from build123d import *

# Parameters (mm, degrees)
SKETCH_1_W          = 14
SKETCH_1_H          = 12
EXTRUDE_1_DEPTH     = 9
FILLET_2_R          = 1
FILLET_3_R          = 1
SKETCH_8_W          = 10
SKETCH_8_H          = 5.607572988
CUT_EXTRUDE_2_DEPTH = 10
SKETCH_9_W          = 10
SKETCH_9_H          = 6
EXTRUDE_3_DEPTH     = 10.1
SKETCH_10_R         = 1.75
CUT_EXTRUDE_3_DEPTH = 0.5
CUT_EXTRUDE_4_DEPTH = 22.740745157
SKETCH_12_W         = 4
SKETCH_12_H         = 5
CUT_EXTRUDE_5_DEPTH = 5
EXTRUDE_5_DEPTH     = 3
SKETCH_17_R         = 5
EXTRUDE_6_DEPTH     = 7
SKETCH_14_R         = 3.5
SKETCH_14_R_2       = 3
EXTRUDE_7_DEPTH     = 10
FILLET_5_R          = 0.5
CUT_EXTRUDE_START   = -5
SKETCH_18_R         = 3
CUT_EXTRUDE_7_DEPTH = 5
FILLET_6_R          = 0.5


# Some blends are built 0.0001 mm under size
with BuildPart() as part:
    # 草图1 → 凸台-拉伸1 (new body)
    with BuildSketch(Plane(origin=(0, 0, 0), x_dir=(1, 0, 0), z_dir=(0, 1, 0))):
        with Locations((7, 6)):
            Rectangle(SKETCH_1_W, SKETCH_1_H)
    extrude(amount=EXTRUDE_1_DEPTH)

    # 圆角2
    fillet_2_edges = [part.edges().sort_by_distance(p)[0] for p in [
        (14, 9, -6),
        (7, 9, -12),
        (0, 9, -6),
        (7, 9, 0),
    ]]
    fillet(fillet_2_edges, radius=FILLET_2_R)

    # 草图4 → 放样1 section 0
    with BuildSketch(Plane.XZ):
        with BuildLine():
            Line((0, 0), (14, 0))
            Line((14, 0), (14, -12))
            Line((14, -12), (0, -12))
            Line((0, -12), (0, 0))
        make_face()
    # 草图5 → 放样1 section 1
    with BuildSketch(Plane(origin=(0, -11, 0), x_dir=(-1, 0, 0), z_dir=(0, -1, 0))):
        with BuildLine():
            Line((-2, 1), (-12, 1))
            Line((-12, 1), (-12, 11))
            Line((-12, 11), (-2, 11))
            Line((-2, 11), (-2, 1))
        make_face()
    loft()

    # 圆角3
    # the kernel refuses this fillet: 1 mm, written as the material it takes off along each edge
    with BuildSketch(Plane(origin=(14.438278825, 2.410533539, -12.219139413), x_dir=(0.015936381457793344, 0.08765009801785527, 0.9960238411119947), z_dir=(-0.1781741612749496, -0.9799578870122228, 0.0890870806374748)), Plane(origin=(14.438278825, 2.410533539, 0.219139413), x_dir=(-0.9839989676081822, 0.17744243678180333, 0.016131130616527562), z_dir=(-0.1781741612749496, -0.9799578870122228, -0.08908708063747467))) as fillet_3_piece_1:
        with BuildLine():
            CenterArc((FILLET_3_R * 0.983933522321, FILLET_3_R), FILLET_3_R, 180.927975892, 89.072024108)
            Line((-FILLET_3_R * 0.0159353215369, FILLET_3_R * 0.983804473396), (0, 0))
            Line((0, 0), (FILLET_3_R * 0.983933522321, 0))
        make_face()
    extrude(amount=16.144639772, mode=Mode.SUBTRACT)
    with BuildSketch(Plane(origin=(-0.438278825, 2.410533539, -12.219139413), x_dir=(-0.015936381457791863, 0.08765009801785537, 0.9960238411119947), z_dir=(0.1781741612749496, -0.9799578870122228, 0.08908708063747463)), Plane(origin=(-0.438278825, 2.410533539, 0.219139413), x_dir=(0.9839989676081822, 0.17744243678180333, 0.016131130616527607), z_dir=(0.1781741612749496, -0.9799578870122228, -0.0890870806374748))) as fillet_3_piece_2:
        with BuildLine():
            CenterArc((FILLET_3_R * 0.983933522321, -FILLET_3_R), FILLET_3_R, 90, 89.072024108)
            Line((-FILLET_3_R * 0.0159353215369, -FILLET_3_R * 0.983804473396), (0, 0))
            Line((0, 0), (FILLET_3_R * 0.983933522321, 0))
        make_face()
    extrude(amount=16.144639772, mode=Mode.SUBTRACT)

    # 草图8 → 切除-拉伸2 (cut)
    with BuildSketch(Plane(origin=(0, 0, -12), x_dir=(-1, 0, 0), z_dir=(0, 0, -1))):
        with Locations((-7, 10.303786494)):
            Rectangle(SKETCH_8_W, SKETCH_8_H)
    extrude(amount=-CUT_EXTRUDE_2_DEPTH, mode=Mode.SUBTRACT)

    # 草图9 → 凸台-拉伸3 (add)
    with BuildSketch(Plane(origin=(0, 0, -2), x_dir=(-1, 0, 0), z_dir=(0, 0, -1))):
        with Locations((-7, 10.5)):
            Rectangle(SKETCH_9_W, SKETCH_9_H)
    extrude(amount=EXTRUDE_3_DEPTH)

    # 草图10 → 切除-拉伸3 (cut)
    with BuildSketch(Plane(origin=(0, 0, -12.1), x_dir=(-1, 0, 0), z_dir=(0, 0, -1))):
        with Locations((-4.5, 10)):
            Circle(SKETCH_10_R)
        with Locations((-9.5, 10)):
            Circle(SKETCH_10_R)
    extrude(amount=-CUT_EXTRUDE_3_DEPTH, mode=Mode.SUBTRACT)

    # 草图11 → 切除-拉伸4 (cut, through all)
    with BuildSketch(Plane.ZY.offset(-2)):
        Polygon((-12.1, 12.5), (-12.1, 13.5), (-9.1, 13.5), align=None)
    extrude(amount=-CUT_EXTRUDE_4_DEPTH, mode=Mode.SUBTRACT)

    # 草图12 → 切除-拉伸5 (cut)
    with BuildSketch(Plane(origin=(0, 13.5, 0), x_dir=(1, 0, 0), z_dir=(0, 1, 0))):
        with Locations((4.5, 5.1)):
            Rectangle(SKETCH_12_W, SKETCH_12_H)
        with Locations((9.5, 5.1)):
            Rectangle(SKETCH_12_W, SKETCH_12_H)
    extrude(amount=-CUT_EXTRUDE_5_DEPTH, mode=Mode.SUBTRACT)

    # 草图15 → 凸台-拉伸5 (add)
    with BuildSketch(Plane.XZ.offset(11)):
        with BuildLine():
            Line((6.95, -5.251668523), (6.95, -6.748331477))
            ThreePointArc((6.95, -6.748331477), (6.25, -6), (6.95, -5.251668523))
        make_face()
        with BuildLine():
            Line((7.05, -5.251668523), (7.05, -6.748331477))
            ThreePointArc((7.05, -6.748331477), (7.75, -6), (7.05, -5.251668523))
        make_face()
    extrude(amount=EXTRUDE_5_DEPTH)

    # 草图17 → 凸台-拉伸6 (add)
    with BuildSketch(Plane.XZ.offset(11)):
        with Locations(Location((7, -6, 0), (0, 0, 270))):
            Circle(SKETCH_17_R)
    extrude(amount=EXTRUDE_6_DEPTH)

    # 草图14 → 凸台-拉伸7 (add)
    with BuildSketch(Plane.XZ.offset(11)):
        with Locations(Location((7, -6, 0), (0, 0, 270))):
            Circle(SKETCH_14_R)
        with Locations(Location((7, -6, 0), (0, 0, 270))):
            Circle(SKETCH_14_R_2, mode=Mode.SUBTRACT)
    extrude(amount=EXTRUDE_7_DEPTH)

    # 圆角5
    fillet_5_edges = [part.edges().sort_by_distance(p)[0] for p in [
        (7, -21, -2.5),
    ]]
    fillet(fillet_5_edges, radius=FILLET_5_R - 0.0001)  # a hair under: the kernel refuses the full size

    # 草图18 → 切除-拉伸7 (cut)
    with BuildSketch(Plane.XZ.offset(18).offset(CUT_EXTRUDE_START)):
        with Locations(Location((7, -6, 0), (0, 0, 270))):
            Circle(SKETCH_18_R)
        with BuildLine():
            Line((6.357738371, -5.9), (7.642261629, -5.9))
            ThreePointArc((7.642261629, -5.9), (7, -5.35), (6.357738371, -5.9))
        make_face(mode=Mode.SUBTRACT)
        with BuildLine():
            Line((6.357738371, -6.1), (7.642261629, -6.1))
            ThreePointArc((7.642261629, -6.1), (7, -6.65), (6.357738371, -6.1))
        make_face(mode=Mode.SUBTRACT)
    extrude(amount=CUT_EXTRUDE_7_DEPTH, mode=Mode.SUBTRACT)

    # 圆角6
    fillet_6_edges = [part.edges().sort_by_distance(p)[0] for p in [
        (7, -18, -5.35),
        (7, -18, -6.65),
    ]]
    fillet(fillet_6_edges, radius=FILLET_6_R)


solid = part.part
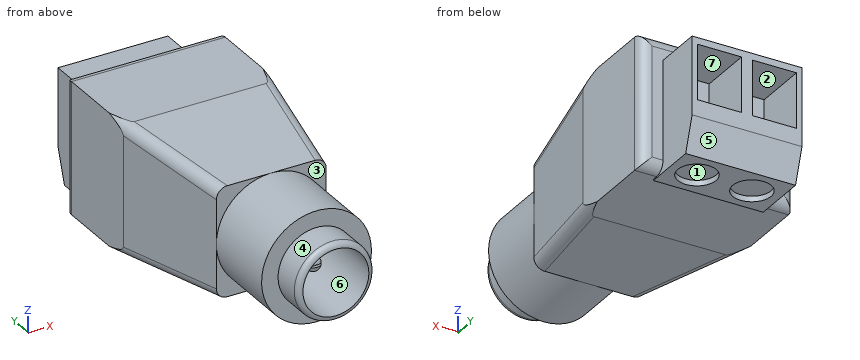
CAD build for the part. Positions are in the model's coordinates, mm. Face numbers are marked on the shaded views. A direction names the side the tool comes from. Coordinates: 2 decimals unless noted, no trailing zeros. Write each loop counter-clockwise with the first axis right and the second up, starting at its lowest first coordinate (ties: lowest second). Pieces come first, ordered by that corner, then holes. Notation, with made-up numbers: M 12,-27.75 L 67,-27.75 A24 cw 67,9.25 Z; hole C -19,-40 d11. An arc over 180 degrees is marked long. Answer as a JSON object with one key per item and string values. Group by question number.
1) Saw through at A-A (y = 10). Write the cut outline in (x, z).
2) Wall check: line 1 (Z direction, x = 4.25, y = 9.5); line 2 (Y direction, x = 3, z = -1.75); line 3 (Z direction, x = 9.25, y = 0.5). Give the ranges that are in metal, low to high. Write a range as from..to.
3) Mould opens along X. For the marked faces 4, 5, 6 and 7 say: +X half, -X half, draft (parallel to the pull), parting line (faces both ways), or undercut.
4) Tool access for the marked faces 1, 2 and 3: list every direction of +Z, -Z, +X, -X, +Y, -Y with a clear straight run to the whole face (end or side of a thin tool).
5) Pin check, flat tips, straight feed: pin 1 Ø1.2 at (x, y) = (3.5, 11.5) entering from +Z; pin 2 Ø3 at (x, z) = (8, -5) entering from +Y; pin 3 Ø1 at (x, y) = (7, -14.5) entering from -Z; pin 4 Ø1.4 at (x, y) = (7, -16) entering from +Z. Stop position of each tip, or through.
Values follow:
{
 "1": {"outline": "M 2,-12.1 L 2.75,-12.1 L 2.75,-11.6 L 6.25,-11.6 L 6.25,-12.1 L 7.75,-12.1 L 7.75,-11.6 L 11.25,-11.6 L 11.25,-12.1 L 12,-12.1 L 12,-2 L 2,-2 Z; hole M 2.5,-7.6 L 6.5,-7.6 L 6.5,-2.6 L 2.5,-2.6 Z; hole M 7.5,-7.6 L 11.5,-7.6 L 11.5,-2.6 L 7.5,-2.6 Z"},
 "2": {"line 1": "z = -11.6..-7.6, -2.6..-2", "line 2": "y = -11..9", "line 3": "z = -12..0"},
 "3": {"face 4": "parting line", "face 5": "draft", "face 6": "undercut", "face 7": "undercut"},
 "4": {"face 1": "-Z", "face 2": "+Y", "face 3": "+Z, +X, -Y"},
 "5": {"pin 1": "stops at z = -2", "pin 2": "stops at y = 13.5", "pin 3": "stops at z = -11", "pin 4": "stops at z = -1"}
}
